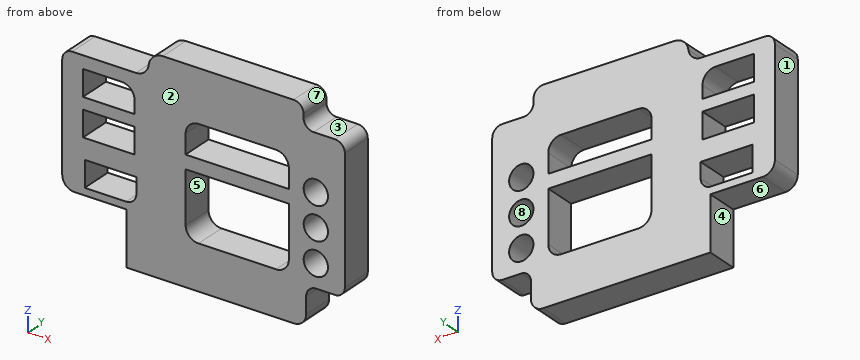
```python
from build123d import *

# Parameters (mm, degrees)
F0_W     = 40
F0_H     = 20
F0_R     = 9.420461
F1_DEPTH = 25
F2_R     = 11.105382
F3_R     = 9.415433
F4_R     = 7.725483
F5_R     = 7.966905


with BuildPart() as f1:
    # F0 (on Front) → F1 (new body)
    with BuildSketch(Plane.XZ):
        with BuildLine():
            Line((-62.390121, 74.47072), (-119.498074, 74.47072))
            Line((-119.498074, 74.47072), (-119.498074, -25.52928))
            Line((-119.498074, -25.52928), (-69.498074, -25.52928))
            Line((-69.498074, -25.52928), (-69.498074, -67.146567))
            Line((-69.498074, -67.146567), (69.608342, -67.146567))
            Line((69.608342, -67.146567), (69.608342, -36.997778))
            Line((69.608342, -36.997778), (99.608342, -36.997778))
            Line((99.608342, -36.997778), (99.608342, 74.47072))
            Line((99.608342, 74.47072), (67.609879, 74.47072))
            Line((67.609879, 74.47072), (67.609879, 92.853433))
            Line((67.609879, 92.853433), (-52.390121, 92.853433))
            Line((-52.390121, 92.853433), (-52.390121, 84.47072))
            ThreePointArc((-52.390121, 84.47072), (-55.319053, 77.399652), (-62.390121, 74.47072))
        make_face()
        with Locations((-81.99026, -10)):
            Rectangle(F0_W, F0_H, mode=Mode.SUBTRACT)
        with BuildLine():
            Line((-23.836674, -22.738976), (-23.836674, 17.261024))
            Line((-23.836674, 17.261024), (56.163326, 17.261024))
            Line((56.163326, 17.261024), (56.163326, -22.738976))
            ThreePointArc((56.163326, -22.738976), (53.234394, -29.810044), (46.163326, -32.738976))
            Line((46.163326, -32.738976), (-13.836674, -32.738976))
            ThreePointArc((-13.836674, -32.738976), (-20.907742, -29.810044), (-23.836674, -22.738976))
        make_face(mode=Mode.SUBTRACT)
        with Locations((77.09389, -18.98604)):
            Circle(F0_R, mode=Mode.SUBTRACT)
        with Locations((77.09389, 6.41396)):
            Circle(F0_R, mode=Mode.SUBTRACT)
        with Locations((-83.39401, 25.578797)):
            Rectangle(F0_W, F0_H, mode=Mode.SUBTRACT)
        with BuildLine():
            Line((-103.39401, 44.666162), (-103.39401, 64.666162))
            Line((-103.39401, 64.666162), (-73.39401, 64.666162))
            ThreePointArc((-73.39401, 64.666162), (-66.322942, 61.73723), (-63.39401, 54.666162))
            Line((-63.39401, 54.666162), (-63.39401, 44.666162))
            Line((-63.39401, 44.666162), (-103.39401, 44.666162))
        make_face(mode=Mode.SUBTRACT)
        with BuildLine():
            Line((56.163326, 27.853433), (-23.836674, 27.853433))
            Line((-23.836674, 27.853433), (-23.836674, 42.853433))
            ThreePointArc((-23.836674, 42.853433), (-20.907742, 49.924501), (-13.836674, 52.853433))
            Line((-13.836674, 52.853433), (46.163326, 52.853433))
            ThreePointArc((46.163326, 52.853433), (53.234394, 49.924501), (56.163326, 42.853433))
            Line((56.163326, 42.853433), (56.163326, 27.853433))
        make_face(mode=Mode.SUBTRACT)
        with Locations((77.09389, 31.81396)):
            Circle(F0_R, mode=Mode.SUBTRACT)
    extrude(amount=F1_DEPTH)

    # F2
    f2_edges = [f1.edges().sort_by_distance(p)[0] for p in [
        (-52.390121, -12.5, 92.853433),
    ]]
    fillet(f2_edges, radius=F2_R)

    # F3
    f3_edges = [f1.edges().sort_by_distance(p)[0] for p in [
        (-119.498074, -12.5, -25.52928),
        (69.608342, -12.5, -67.146567),
    ]]
    fillet(f3_edges, radius=F3_R)

    # F4
    f4_edges = [f1.edges().sort_by_distance(p)[0] for p in [
        (67.609879, -12.5, 92.853433),
        (67.609879, -12.5, 74.47072),
        (99.608342, -12.5, 74.47072),
        (-119.498074, -12.5, 74.47072),
        (99.608342, -12.5, -36.997778),
        (69.608342, -12.5, -36.997778),
    ]]
    fillet(f4_edges, radius=F4_R)

    # F5
    f5_edges = [f1.edges().sort_by_distance(p)[0] for p in [
        (-61.99026, -12.5, -20),
    ]]
    fillet(f5_edges, radius=F5_R)


solid = f1.part
```
Design review of the part built by this model. Coordinates are the model's own, in mm. Face numbers are marked on the shaded views. A direction names the side the tool comes from. Give positions to 0.01 mm unless a question says otherwise; leave off trailing zeros. Loops run counter-clockwise (first coordinate to the right, second up) from the corner with the lowest first, then second, coordinate; pieces in that order, holes last. Notation, with made-up numbers: M 47,67 L 53,67 A13 cw 53,75 Z; hole C -13.5,82 d1. An arc over 180 degrees is marked long. Return JSON: item names as keys, results as strings. Group by question number.
Item 1: Mouldability with a two-part tool opening along X and no side actions: class the marked faces 6, 7 and 8 as released by +X, released by -X, zero draft, split by the parting line, or undercut.
Item 2: We need section A-A (x = 20). Give the boundary of the cut face in (y, z).
Item 3: We need section D-D (y = -20). Give the number of separate pieces and of enclosed holes in the cut face, and give its area (3 significant figures).
Item 4: For probe 1 along Z at (x, y) = (-79, -14.5); probe 2 along Z at (x, y) = (-11.5, -20.5); probe 3 along X at (y, z) = (-14.5, 13.5), list the stretches that pass through material, from the lowest coordinate up.
Item 5: We need section B-B (x = 72). Give the boundary of the cut face in (y, z), and give its area (3 significant figures).
Item 6: Insertion check: pin 1 Ø12.5 at (y, z) = (-10, -45) entering from -X; pin 2 Ø10 at (x, y) = (-46, -5.5) entering from +Z; pin 3 Ø12 at (y, z) = (-7, -27.5) entering from -X; pin 4 Ø6.5 at (y, z) = (-16.5, -52.5) entering from +X. Each pin has a flat end and moves straight along its axis. Give the tip position at first contact, or say it passes through.
Item 7: We need section C-C (z = -53.5). Give the boundary of the cut face in (x, y), and give its area (3 significant figures).
Item 8: Tool access review of the marked faces 1, 2, 3, 4 and 5: name each direction out of +Z, -Z, +X, -X, +Y, -Y from which nothing blocks a thin tool from reaching the whole face with its end or side.
Output:
{
 "1": {"face 6": "zero draft", "face 7": "released by +X", "face 8": "undercut"},
 "2": {"outline": "M -25,-67.15 L 0,-67.15 L 0,-32.74 L -25,-32.74 Z; M -25,17.26 L 0,17.26 L 0,27.85 L -25,27.85 Z; M -25,52.85 L 0,52.85 L 0,92.85 L -25,92.85 Z"},
 "3": {"separate pieces": "1", "enclosed holes": "8", "area": "21,100 mm^2"},
 "4": {"probe 1": "z = -25.53 to -20, 0 to 15.58, 35.58 to 44.67, 64.67 to 74.47", "probe 2": "z = -67.15 to -32.74, 17.26 to 27.85, 52.85 to 92.85", "probe 3": "x = -119.5 to -23.84, 56.16 to 70.89, 83.3 to 99.61"},
 "5": {"outline": "M -25,-39.13 L 0,-39.13 L 0,-26.91 L -25,-26.91 Z; M -25,-11.06 L 0,-11.06 L 0,-1.51 L -25,-1.51 Z; M -25,14.34 L 0,14.34 L 0,23.89 L -25,23.89 Z; M -25,39.74 L 0,39.74 L 0,75.23 L -25,75.23 Z", "area": "1,670 mm^2"},
 "6": {"pin 1": "stops at x = -69.5", "pin 2": "stops at z = 92.85", "pin 3": "stops at x = -117.81", "pin 4": "stops at x = 69.61"},
 "7": {"outline": "M -69.5,-25 L 69.61,-25 L 69.61,0 L -69.5,0 Z", "area": "3,480 mm^2"},
 "8": {"face 1": "+Z, -Z, -X, +Y, -Y", "face 2": "+Z, -Z, +X, -X, -Y", "face 3": "+Z, +X, +Y, -Y", "face 4": "-Z, -X, +Y, -Y", "face 5": "+Y, -Y"}
}
